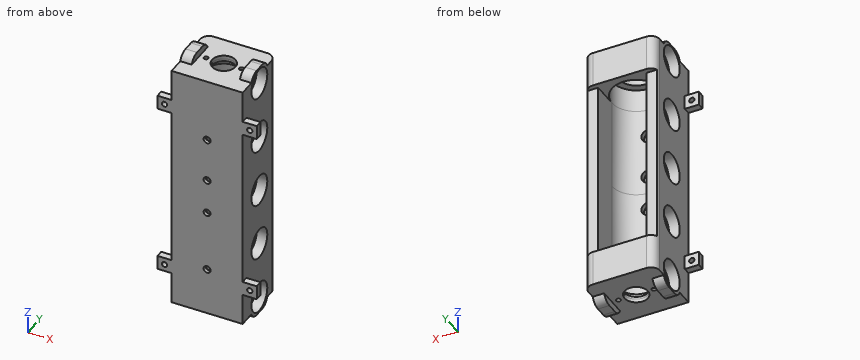
```python
from build123d import *

# Parameters (mm, degrees)
CROQUIS1_R              = 13.7
SALIENTE_EXTRUIR1_DEPTH = 5
CROQUIS2_R              = 9.5
CORTAR_EXTRUIR1_DEPTH   = 3.5
CROQUIS3_R              = 6.8
CORTAR_EXTRUIR2_DEPTH   = 3
SALIENTE_EXTRUIR2_START = 2
CROQUIS4_R              = 13.7
CROQUIS4_R_2            = 6.65
SALIENTE_EXTRUIR2_DEPTH = 2
CROQUIS5_R              = 1.25
CORTAR_EXTRUIR3_DEPTH   = 21.600485431
CROQUIS6_W              = 40.4
CROQUIS6_H              = 36
CROQUIS6_R              = 13.7
SALIENTE_EXTRUIR3_DEPTH = 20
CROQUIS8_W              = 6.5
CROQUIS8_H              = 15
SALIENTE_EXTRUIR5_DEPTH = 51.5
CROQUIS11_W             = 6.5
CROQUIS11_H             = 17.1
SALIENTE_EXTRUIR6_DEPTH = 4
CROQUIS9_R              = 8.55
CORTAR_EXTRUIR4_DEPTH   = 6
REDONDEO1_R             = 5
REDONDEO2_R             = 5
CROQUIS10_R             = 4
CORTAR_EXTRUIR5_DEPTH   = 16
CROQUIS12_R             = 2
CORTAR_EXTRUIR6_DEPTH   = 24
REDONDEO4_R             = 6
REDONDEO5_R             = 6
CROQUIS13_W             = 8
CROQUIS13_H             = 4
SALIENTE_EXTRUIR7_DEPTH = 8
CROQUIS14_R             = 1.5
CORTAR_EXTRUIR7_DEPTH   = 8


with BuildPart() as part:
    # Croquis1 → Saliente-Extruir1 (new body)
    with BuildSketch(Plane.XY):
        Circle(CROQUIS1_R)
        with BuildLine():
            Line((0, 0.75), (7.800197377, 0.75))
            ThreePointArc((7.800197377, 0.75), (10.459785271, 2.369760146), (12.48, 0))
            ThreePointArc((12.48, 0), (10.459785271, -2.369760146), (7.800197377, -0.75))
            Line((7.800197377, -0.75), (0, -0.75))
            Line((0, -0.75), (-7.800197377, -0.75))
            ThreePointArc((-7.800197377, -0.75), (-12.48, 0), (-7.800197377, 0.75))
            Line((-7.800197377, 0.75), (0, 0.75))
        make_face(mode=Mode.SUBTRACT)
    extrude(amount=SALIENTE_EXTRUIR1_DEPTH)

    # Croquis2 → Cortar-Extruir1 (cut)
    with BuildSketch(Plane.XY.offset(5)):
        Circle(CROQUIS2_R)
    extrude(amount=-CORTAR_EXTRUIR1_DEPTH, mode=Mode.SUBTRACT)

    # Croquis3 → Cortar-Extruir2 (cut)
    with BuildSketch(Plane.XY.offset(1.5)):
        Circle(CROQUIS3_R)
    extrude(amount=-CORTAR_EXTRUIR2_DEPTH, mode=Mode.SUBTRACT)

    # Croquis4 → Saliente-Extruir2 (add)
    with BuildSketch(Plane(origin=(0, 0, 0), x_dir=(-1, 0, 0), z_dir=(0, 0, -1)).offset(SALIENTE_EXTRUIR2_START)):
        Circle(CROQUIS4_R)
        Circle(CROQUIS4_R_2, mode=Mode.SUBTRACT)
    extrude(amount=-SALIENTE_EXTRUIR2_DEPTH)

    # Croquis5 → Cortar-Extruir3 (cut, through all)
    with BuildSketch(Plane.XY.offset(5)):
        with Locations((-10.08, 0)):
            Circle(CROQUIS5_R)
        with Locations((10.08, 0)):
            Circle(CROQUIS5_R)
    extrude(amount=-CORTAR_EXTRUIR3_DEPTH, mode=Mode.SUBTRACT)



with BuildPart() as body_2:
    # Croquis6 → Saliente-Extruir3 (new body)
    with BuildSketch(Plane(origin=(0, 0, -2), x_dir=(-1, 0, 0), z_dir=(0, 0, -1))):
        Rectangle(CROQUIS6_W, CROQUIS6_H)
        Circle(CROQUIS6_R, mode=Mode.SUBTRACT)
    extrude(amount=-SALIENTE_EXTRUIR3_DEPTH)

    # Croquis8 → Saliente-Extruir5 (add)
    with BuildSketch(Plane.XY.offset(18)):
        with BuildLine():
            ThreePointArc((13.7, 0), (0, -13.7), (-13.7, 0))
            Line((-13.7, 0), (-20.2, 0))
            Line((-20.2, 0), (-20.2, -18))
            Line((-20.2, -18), (20.2, -18))
            Line((20.2, -18), (20.2, 0))
            Line((20.2, 0), (13.7, 0))
        make_face()
        with Locations((-16.95, 7.5)):
            Rectangle(CROQUIS8_W, CROQUIS8_H)
        with Locations((16.95, 7.5)):
            Rectangle(CROQUIS8_W, CROQUIS8_H)
    extrude(amount=SALIENTE_EXTRUIR5_DEPTH)


with BuildPart() as part_1:
    add(part.part)

    add(body_2.part)  # Saliente-Extruir6 merges body 2
    # Croquis11 → Saliente-Extruir6 (add)
    with BuildSketch(Plane(origin=(0, 0, -2), x_dir=(-1, 0, 0), z_dir=(0, 0, -1))):
        with Locations((-16.95, 0)):
            Rectangle(CROQUIS11_W, CROQUIS11_H)
        with Locations((16.95, 0)):
            Rectangle(CROQUIS11_W, CROQUIS11_H)
    extrude(amount=SALIENTE_EXTRUIR6_DEPTH)


with BuildPart() as body_2_2:
    # Simetría10: mirrored copy
    add(part_1.part.mirror(Plane.XY.offset(69.5)))


with BuildPart() as cortar_extruir4_tool:
    # Croquis9 → Cortar-Extruir4 (new body)
    with BuildSketch(Plane.ZY.offset(20.2)):
        with Locations((3.479126344, 0)):
            Circle(CROQUIS9_R)
        with Locations((36.479126344, 0)):
            Circle(CROQUIS9_R)
        with Locations((69.479126344, 0)):
            Circle(CROQUIS9_R)
        with Locations((102.479126344, 0)):
            Circle(CROQUIS9_R)
        with Locations((135.479126344, 0)):
            Circle(CROQUIS9_R)
    cortar_extruir4 = extrude(amount=-CORTAR_EXTRUIR4_DEPTH)


with BuildPart() as part_2:
    add(part_1.part)

    # Cortar-Extruir4: cut by cortar_extruir4_tool
    add(cortar_extruir4_tool.part, mode=Mode.SUBTRACT)


with BuildPart() as body_2_2_1:
    add(body_2_2.part)

    # Cortar-Extruir4: cut by cortar_extruir4_tool
    add(cortar_extruir4_tool.part, mode=Mode.SUBTRACT)


with BuildPart() as simetr_a11_tool:
    # Simetría11: Cortar-Extruir4 across plane
    add(cortar_extruir4.mirror(Plane(origin=(0, 0, 0), x_dir=(0, 0, 1), z_dir=(1, 0, 0))))


with BuildPart() as part_3:
    add(part_2.part)

    # Simetría11: cut by simetr_a11_tool
    add(simetr_a11_tool.part, mode=Mode.SUBTRACT)

    # Redondeo1
    redondeo1_edges = [part_3.edges().sort_by_distance(p)[0] for p in [
        (20.2, 18, 8),
        (-20.2, 18, 8),
    ]]
    fillet(redondeo1_edges, radius=REDONDEO1_R)


with BuildPart() as body_2_2_2:
    add(body_2_2_1.part)

    # Simetría11: cut by simetr_a11_tool
    add(simetr_a11_tool.part, mode=Mode.SUBTRACT)

    # Redondeo2
    redondeo2_edges = [body_2_2_2.edges().sort_by_distance(p)[0] for p in [
        (20.2, 18, 131),
        (-20.2, 18, 131),
    ]]
    fillet(redondeo2_edges, radius=REDONDEO2_R)


with BuildPart() as cortar_extruir5_tool:
    # Croquis10 → Cortar-Extruir5 (new body)
    with BuildSketch(Plane.XZ):
        with Locations(Location((0, 60, 0), (0, 0, 90))):
            Circle(CROQUIS10_R)
        with Locations(Location((0, 105, 0), (0, 0, 90))):
            Circle(CROQUIS10_R)
        with Locations(Location((0, 80, 0), (0, 0, 90))):
            Circle(CROQUIS10_R)
        with Locations(Location((0, 25, 0), (0, 0, 90))):
            Circle(CROQUIS10_R)
    extrude(amount=CORTAR_EXTRUIR5_DEPTH)


with BuildPart() as part_4:
    add(part_3.part)

    # Cortar-Extruir5: cut by cortar_extruir5_tool
    add(cortar_extruir5_tool.part, mode=Mode.SUBTRACT)


with BuildPart() as body_2_2_3:
    add(body_2_2_2.part)

    # Cortar-Extruir5: cut by cortar_extruir5_tool
    add(cortar_extruir5_tool.part, mode=Mode.SUBTRACT)


with BuildPart() as cortar_extruir6_tool:
    # Croquis12 → Cortar-Extruir6 (new body)
    with BuildSketch(Plane.XZ):
        with Locations(Location((0, 60, 0), (0, 0, 270))):
            Circle(CROQUIS12_R)
        with Locations(Location((0, 105, 0), (0, 0, 270))):
            Circle(CROQUIS12_R)
        with Locations(Location((0, 80, 0), (0, 0, 270))):
            Circle(CROQUIS12_R)
        with Locations(Location((0, 25, 0), (0, 0, 270))):
            Circle(CROQUIS12_R)
    extrude(amount=CORTAR_EXTRUIR6_DEPTH)


with BuildPart() as part_5:
    add(part_4.part)

    # Cortar-Extruir6: cut by cortar_extruir6_tool
    add(cortar_extruir6_tool.part, mode=Mode.SUBTRACT)

    # Redondeo5
    # the kernel refuses this fillet: 6 mm, written as the material it takes off along each edge
    with BuildSketch(Plane(origin=(-34.342135624, -8.55, -6), x_dir=(0, 0, 1), z_dir=(1, 0, 0)), Plane(origin=(0.442135624, 8.55, -6), x_dir=(0, 0, 1), z_dir=(-1, 0, 0)), Plane(origin=(34.342135624, 8.55, -6), x_dir=(0, 0, 1), z_dir=(-1, 0, 0))) as redondeo5_piece_1:
        with BuildLine():
            CenterArc((6, -5.656854249), REDONDEO5_R, 109.471220634, 70.528779366)
            Line((0, -5.656854249), (-0.12, -5.656854249))
            Line((-0.12, -5.656854249), (-0.12, 0))
            Line((-0.12, 0), (0, 0.12))
            ThreePointArc((0, 0.12), (2, 0.12), (3.96, 0.113137085))
            Line((3.96, 0.113137085), (4, 0))
        make_face()
    extrude(amount=34.784271247, mode=Mode.SUBTRACT)
    with BuildSketch(Plane(origin=(-0.442135624, -8.55, -6), x_dir=(0, 1, 0), z_dir=(1, 0, 0))) as redondeo5_piece_2:
        with BuildLine():
            CenterArc((5.656854249, 6), REDONDEO5_R, 199.471220634, 70.528779366)
            Line((0, 4), (-0.113137085, 3.96))
            ThreePointArc((-0.113137085, 3.96), (-0.12, 2), (-0.12, 0))
            Line((-0.12, 0), (0, -0.12))
            Line((0, -0.12), (5.656854249, -0.12))
            Line((5.656854249, -0.12), (5.656854249, 0))
        make_face()
    extrude(amount=34.784271247, mode=Mode.SUBTRACT)



with BuildPart() as body_2_2_4:
    add(body_2_2_3.part)

    # Cortar-Extruir6: cut by cortar_extruir6_tool
    add(cortar_extruir6_tool.part, mode=Mode.SUBTRACT)

    # Redondeo4
    # the kernel refuses this fillet: 6 mm, written as the material it takes off along each edge
    with BuildSketch(Plane(origin=(-34.342135624, -8.55, 145), x_dir=(0, 0, -1), z_dir=(1, 0, 0)), Plane(origin=(0.442135624, 8.55, 145), x_dir=(0, 0, -1), z_dir=(-1, 0, 0)), Plane(origin=(-0.442135624, -8.55, 145), x_dir=(0, 0, -1), z_dir=(1, 0, 0)), Plane(origin=(34.342135624, 8.55, 145), x_dir=(0, 0, -1), z_dir=(-1, 0, 0))) as redondeo4_piece_1:
        with BuildLine():
            CenterArc((6, 5.656854249), REDONDEO4_R, 180, 70.528779366)
            Line((0, 5.656854249), (-0.12, 5.656854249))
            Line((-0.12, 5.656854249), (-0.12, 0))
            Line((-0.12, 0), (0, -0.12))
            ThreePointArc((0, -0.12), (2, -0.12), (3.96, -0.113137085))
            Line((3.96, -0.113137085), (4, 0))
        make_face()
    extrude(amount=34.784271247, mode=Mode.SUBTRACT)


with BuildPart() as part_6:
    add(part_5.part)

    add(body_2_2_4.part)  # Saliente-Extruir7 merges body 2 2
    # Croquis13 → Saliente-Extruir7 (add)
    with BuildSketch(Plane.ZY.offset(20.2)):
        with Locations((19.979126344, -16)):
            Rectangle(CROQUIS13_W, CROQUIS13_H)
        with Locations((118.979126344, -16)):
            Rectangle(CROQUIS13_W, CROQUIS13_H)
    saliente_extruir7 = extrude(amount=SALIENTE_EXTRUIR7_DEPTH)

    # Croquis14 → Cortar-Extruir7 (cut)
    with BuildSketch(Plane(origin=(0, -14, 0), x_dir=(1, 0, 0), z_dir=(0, 1, 0))):
        with Locations(Location((-24.2, -19.979126344, 0), (0, 0, 270))):
            Circle(CROQUIS14_R)
        with Locations(Location((-24.2, -119.020873656, 0), (0, 0, 90))):
            Circle(CROQUIS14_R)
    cortar_extruir7 = extrude(amount=-CORTAR_EXTRUIR7_DEPTH, mode=Mode.SUBTRACT)

    # Simetría12: Saliente-Extruir7, Cortar-Extruir7 across plane
    add(saliente_extruir7.mirror(Plane(origin=(0, 0, 0), x_dir=(0, 0, 1), z_dir=(1, 0, 0))))
    add(cortar_extruir7.mirror(Plane(origin=(0, 0, 0), x_dir=(0, 0, 1), z_dir=(1, 0, 0))), mode=Mode.SUBTRACT)


solid = part_6.part
```
The listing builds one solid part. Answer for the finished solid, in the listing's coordinates (mm). Coordinates: 2 decimals unless noted, no trailing zeros. Loops run counter-clockwise (first coordinate to the right, second up) from the corner with the lowest first, then second, coordinate; pieces in that order, holes last. Notation, with made-up numbers: (55.5, -20.5) - (70.5, -20.5) arc R19 cw to (70.5, 4.5) - close; hole circle Ø7 at (-35.75, 18). An arc over 180 degrees is marked (long way). Use a Markdown table: item, result. Add a question column.
1) The part is cut by section B-B, the plane z = 80. Give the vertices of the cut face in (x, y), and give its area (3 significant figures).
2) Find the intervals of material crossed by line 1 (X direction, y = 4, z = 81); line 2 (Y direction, x = 0, z = 126); line 3 (Z direction, x = -2.5, y = 12), in increasing order.
3) The part is cut by section A-A, the plane x = -24.2. Give the vertices of the cut face in (y, z), and give its area (3 significant figures).
4) The part is cut by section D-D, the plane z = 33.5. Give the vertices of the cut face in (x, y).
5) Given pin 1 (1.5 mm diameter, centred on x = 19, y = -13, fed in from +Z); pin 2 (3 mm diameter, centred on x = 15.5, z = 61, fed in from +Y); pin 3 (10 mm diameter, centred on y = -8, z = 80.5, fed in from +X); pin 4 (1 mm diameter, centred on x = -21, y = -1.5, fed in from +Z), each flat-ended and moving along its own axis, determine where each tip first touches the part or whether it passes through.
6) The part is cut by section C-C, the plane x = 0. State how many separate pieces and enclosed holes the cut face has, and give its area (3 significant figures).
Here are the results:
| question | item | result |
|---|---|---|
| 1 | outline | (-20.2, -18) - (-2, -18) - (-2, -16) - (-4, -16) - (-4, -13.1) arc R13.7 cw to (-13.7, 0) - (-13.7, 15) - (-19.78, 15) arc R5 ccw to (-20.2, 13) - close; (2, -18) - (20.2, -18) - (20.2, 13) arc R5 ccw to (19.78, 15) - (13.7, 15) - (13.7, 0) arc R13.7 cw to (4, -13.1) - (4, -16) - (2, -16) - close |
| 1 | area | 599 mm^2 |
| 2 | line 1 | x = -20.2 to -13.7, 13.7 to 20.2 |
| 2 | line 2 | y = -18 to -13.7, 13.7 to 18 |
| 2 | line 3 | z = -2 to 5, 134 to 141 |
| 3 | outline | (-18, 15.98) - (-14, 15.98) - (-14, 18.48) - (-18, 18.48) - close; (-18, 21.48) - (-14, 21.48) - (-14, 23.98) - (-18, 23.98) - close; (-18, 114.98) - (-14, 114.98) - (-14, 117.52) - (-18, 117.52) - close; (-18, 120.52) - (-14, 120.52) - (-14, 122.98) - (-18, 122.98) - close |
| 3 | area | 40.0 mm^2 |
| 4 | outline | (-20.2, -18) - (20.2, -18) - (20.2, -8.01) - (14.2, -8.01) - (14.2, 8.01) - (20.2, 8.01) - (20.2, 13) arc R5 ccw to (19.78, 15) - (13.7, 15) - (13.7, 0) arc R13.7 cw to (-13.7, 0) - (-13.7, 15) - (-19.78, 15) arc R5 ccw to (-20.2, 13) - (-20.2, 8.01) - (-14.2, 8.01) - (-14.2, -8.01) - (-20.2, -8.01) - close |
| 5 | pin 1 | stops at z = 141 |
| 5 | pin 2 | stops at y = 15 |
| 5 | pin 3 | stops at x = 20.2 |
| 5 | pin 4 | passes through |
| 6 | separate pieces | 7 |
| 6 | enclosed holes | 0 |
| 6 | area | 838 mm^2 |
